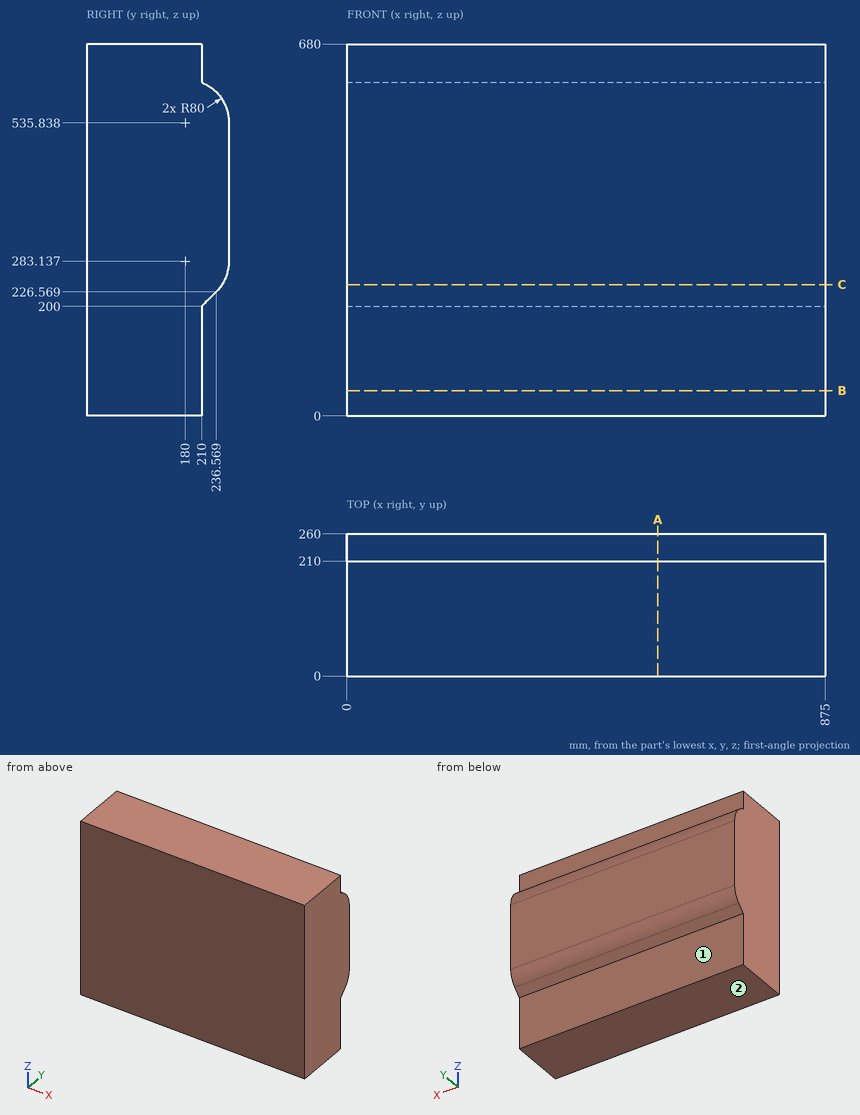
Design review of the part shown in the three views and the two pictorial views. Dimensions are in mm from the part's minimum x, y and z. A direction names the side the tool comes from. Round coordinates to 2 decimals unless told otherwise and drop trailing zeros. Write each loop counter-clockwise with the first axis right and the second up, starting at its lowest first coordinate (ties: lowest second). Pieces come first, ordered by that corner, then holes. Notation, with made-up numbers: M 68,-24 L 100,-24 A22 ccw 100,-3 Z; hole C -11,-18 d6. An arc over 180 degrees is marked long. One line per item, written item: value. Start each with the question number.
1. Take a section at A-A on x = 569. State the section outline as (y, z) points, then the cut area to 3 significant figures.
2. Take a section at C-C on z = 240. State the section outline as (x, y) points.
3. To check wall thickness, follow probe 1 along Y at (x, z) = (514, 625); probe 2 along Y at (x, z) = (804.5, 207); probe 3 along Z at (x, y) = (438.5, 230). State the ranges of each line that lie inside material, in increasing order. Write a range as from..to.
4. For the marked faces 1 and 2, list the 3-axis set-ups (+Z, -Z, +X, -X, +Y, -Y) from which the entire face can be reached by the end or side of a thin tool; tool diameter is ignored.
5. Take a section at B-B on z = 46. State the section outline as (x, y) points, then the cut area to 3 significant figures.
6. Clearance check with flat-ended pins moving along their axes: P1, Ø12, axis at x = 191, z = 160.5, coming from the +Y side; P2, Ø8, axis at x = 129, z = 570.5, coming from the +Y side; P3, Ø6, axis at x = 623.5, z = 588, coming from the +Y side. State where each tip first meets the part, or that it passes through.
Computed:
1. outline: M 0,0 L 210,0 L 210,200 L 236.57,226.57 A80 ccw 260,283.14 L 260,535.84 A80 ccw 210,610 L 210,680 L 0,680 Z
1. area: 161,000 mm²
2. outline: M 0,0 L 875,0 L 875,247.37 L 0,247.37 Z
3. probe 1: y = 0..210
3. probe 2: y = 0..217
3. probe 3: z = 220..598.29
4. face 1: -Z, +X, -X, +Y
4. face 2: -Z, +X, -X, +Y, -Y
5. outline: M 0,0 L 875,0 L 875,210 L 0,210 Z
5. area: 184,000 mm²
6. P1: stops at y = 210
6. P2: stops at y = 253.89
6. P3: stops at y = 243.11
